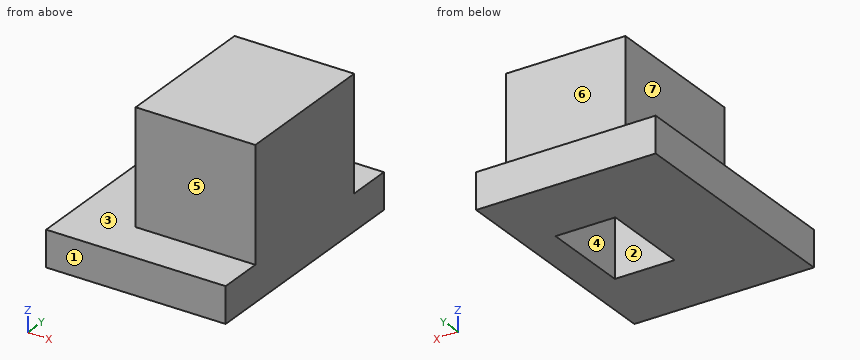
```python
from build123d import *

# Parameters (mm, degrees)
SKETCH_1_W      = 4
SKETCH_1_H      = 5
SKETCH_1_W_2    = 2
SKETCH_1_H_2    = 3
EXTRUDE_1_DEPTH = 4
EXTRUDE_2_DEPTH = 1.2
SKETCH_3_W      = 4
SKETCH_3_H      = 5
EXTRUDE_3_DEPTH = 1


with BuildPart() as part:
    # 草图1 → 凸台-拉伸1 (new body)
    with BuildSketch(Plane.XY):
        with Locations((1, 1.5)):
            Rectangle(SKETCH_1_W, SKETCH_1_H)
        with Locations((1, 1.5)):
            Rectangle(SKETCH_1_W_2, SKETCH_1_H_2, mode=Mode.SUBTRACT)
    extrude(amount=EXTRUDE_1_DEPTH)

    # 草图2 → 凸台-拉伸2 (add)
    with BuildSketch(Plane(origin=(0, 0, 0), x_dir=(-1, 0, 0), z_dir=(0, 0, -1))):
        Polygon((-3, 4), (1, 4), (1, -1), (-3, -1), (-3, -2.5), (3, -2.5), (3, 5.5), (-3, 5.5), align=None)
    extrude(amount=-EXTRUDE_2_DEPTH)

    # 草图3 → 凸台-拉伸3 (add)
    with BuildSketch(Plane.XY.offset(4)):
        with Locations((1, 1.5)):
            Rectangle(SKETCH_3_W, SKETCH_3_H)
    extrude(amount=EXTRUDE_3_DEPTH)


solid = part.part
```
Source: CAD feature listing. Evaluate the final solid. Frame: model axes, mm. Face numbers are marked on the shaded views. A direction names the side the tool comes from. Round coordinates to 2 decimals unless told otherwise and drop trailing zeros. Loops run counter-clockwise (first coordinate to the right, second up) from the corner with the lowest first, then second, coordinate; pieces in that order, holes last. Notation, with made-up numbers: (74.25, -13) - (106.25, -13) arc R34 cw to (106.25, 18) - close; hole circle Ø3 at (25, 42). An arc over 180 degrees is marked (long way). Use CSV: the item, a comma, the result in double quotes.
Q1. Section query D-D, the plane z = 0.5. Output: boundary loops of the cut face in (x, y), then the cut area to 3 significant figures.
Reported:
outline,"(-3, -2.5) - (3, -2.5) - (3, 5.5) - (-3, 5.5) - close; hole (0, 0) - (2, 0) - (2, 3) - (0, 3) - close"
area,"42.0 mm^2"
Q2. Pin query (flat end, axial travel): pin 1 Ø1.5 at (y, z) = (4, 3) entering from -X; pin 2 Ø1.6 at (x, z) = (0.5, 2.5) entering from -Y; pin 3 Ø3 at (x, z) = (1, 3) entering from +Y. Return the tip coordinate at first contact, or that it passes through.
Reported:
pin 1,"x = -1"
pin 2,"y = -1"
pin 3,"y = 4"
Q3. Section query B-B, the plane y = 2.5. Output: boundary loops of the cut face in (x, z).
Reported:
outline,"(-3, 0) - (0, 0) - (0, 4) - (2, 4) - (2, 0) - (3, 0) - (3, 5) - (-1, 5) - (-1, 1.2) - (-3, 1.2) - close"
Q4. Mould query, pull axis Y, two halves, no side actions, for the marked faces 1, 2, 3 and 4. Classes: pulls with the +Y half, pulls with the -Y half, needs draft (parallel to the pull), parting line crosses it, or undercut.
Reported:
face 1,"pulls with the -Y half"
face 2,"undercut"
face 3,"needs draft"
face 4,"undercut"
Q5. Ray query, line 1 along Y through (x, z) = (1.05, 3.7); line 2 along X through (y, z) = (2.25, 1.6); line 3 along X through (y, z) = (1, 0.85). Return the intervals inside material, ascending.
Reported:
line 1,"-1 to 0, 3 to 4"
line 2,"-1 to 0, 2 to 3"
line 3,"-3 to 0, 2 to 3"
Q6. Section query A-A, the plane z = 2.9. Output: boundary loops of the cut face in (x, y).
Reported:
outline,"(-1, -1) - (3, -1) - (3, 4) - (-1, 4) - close; hole (0, 0) - (2, 0) - (2, 3) - (0, 3) - close"
Q7. Section query C-C, the plane x = 2.15. Output: boundary loops of the cut face in (y, z), then the cut area to 3 significant figures.
Reported:
outline,"(-2.5, 0) - (5.5, 0) - (5.5, 1.2) - (4, 1.2) - (4, 5) - (-1, 5) - (-1, 1.2) - (-2.5, 1.2) - close"
area,"28.6 mm^2"
Q8. Reachability of the marked faces 5, 6 and 7 from +Z, -Z, +X, -X, +Y, -Y: full face, straight path, thin tool, end or side. Return the list, or none.
Reported:
face 5,"+Z, +X, -X, -Y"
face 6,"+Z, +X, -X, +Y"
face 7,"+Z, -X, +Y, -Y"
